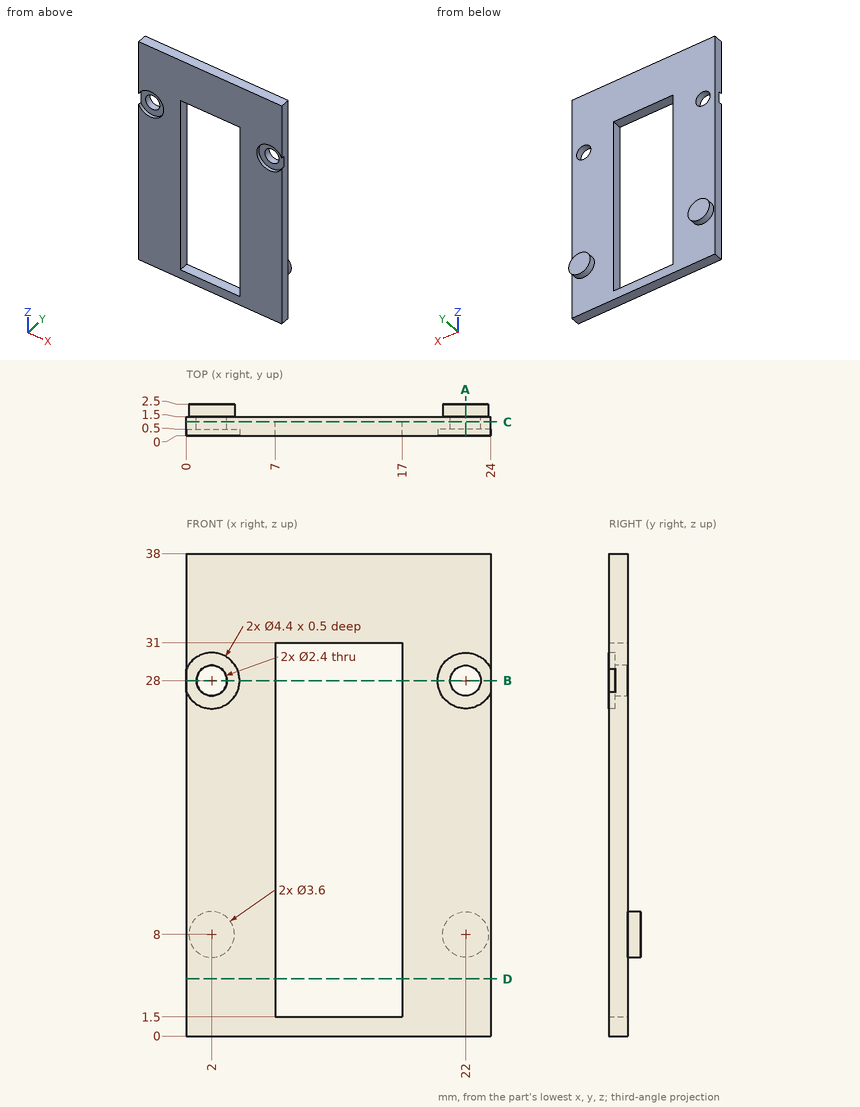
Design review of the part shown in the three views and the two pictorial views. Dimensions are in mm from the part's minimum x, y and z. Give positions to 0.01 mm unless a question says otherwise; leave off trailing zeros. Loops run counter-clockwise (first coordinate to the right, second up) from the corner with the lowest first, then second, coordinate; pieces in that order, holes last. Notation, with made-up numbers: (-32, 54) -> (20, 54) arc R27 ccw to (20, 87) -> close; hole circle Ø6 at (-11.75, 79). An arc over 180 degrees is marked (long way). Answer as a JSON object with one key per item and string values. Group by question number.
Q1. Wall thickness on line 1 along Z through (x, y) = (2, 0.4); line 2 along Z through (x, y) = (12.75, 0.1); line 3 along X through (y, z) = (0.4, 2): over which ranges is each line inside the solid? List them lowest first.
Q2. Take a section at D-D (z = 4.5). Write out the cut boundary in (x, y).
Q3. Insertion check: pin 1 (5 mm diameter, centred on x = 2, z = 28, fed in from +Y); pin 2 (1.2 mm diameter, centred on x = 12.5, y = 1, fed in from -Z); pin 3 (1.3 mm diameter, centred on x = 21.5, z = 27.5, fed in from -Y). Each pin has a flat end and moves straight along its axis. Give the tip position at first contact, or say it passes through.
Q4. Take a section at B-B (z = 28). Write out the cut boundary in (x, y), plus the area to 3 significant figures.
Q5. Take a section at C-C (y = 1.1). Write out the cut boundary in (x, z), plus the area to 3 significant figures.
Q6. Take a section at A-A (x = 22). Write out the cut boundary in (y, z).
Answer below:
{
 "1": {"line 1": "z = 0 to 25.8, 30.2 to 38", "line 2": "z = 0 to 1.5, 31 to 38", "line 3": "x = 0 to 7, 17 to 24"},
 "2": {"outline": "(0, 0) -> (7, 0) -> (7, 1.5) -> (0, 1.5) -> close; (17, 0) -> (24, 0) -> (24, 1.5) -> (17, 1.5) -> close"},
 "3": {"pin 1": "stops at y = 1.5", "pin 2": "stops at z = 0", "pin 3": "stops at y = 0.5"},
 "4": {"outline": "(0, 0.5) -> (0.8, 0.5) -> (0.8, 1.5) -> (0, 1.5) -> close; (3.2, 0.5) -> (4.2, 0.5) -> (4.2, 0) -> (7, 0) -> (7, 1.5) -> (3.2, 1.5) -> close; (17, 0) -> (19.8, 0) -> (19.8, 0.5) -> (20.8, 0.5) -> (20.8, 1.5) -> (17, 1.5) -> close; (23.2, 0.5) -> (24, 0.5) -> (24, 1.5) -> (23.2, 1.5) -> close", "area": "12.0 mm2"},
 "5": {"outline": "(0, 0) -> (24, 0) -> (24, 38) -> (0, 38) -> close; hole circle Ø2.4 at (2, 28); hole (7, 1.5) -> (17, 1.5) -> (17, 31) -> (7, 31) -> close; hole circle Ø2.4 at (22, 28)", "area": "608 mm2"},
 "6": {"outline": "(0, 0) -> (1.5, 0) -> (1.5, 6.2) -> (2.5, 6.2) -> (2.5, 9.8) -> (1.5, 9.8) -> (1.5, 26.8) -> (0.5, 26.8) -> (0.5, 25.8) -> (0, 25.8) -> close; (0, 30.2) -> (0.5, 30.2) -> (0.5, 29.2) -> (1.5, 29.2) -> (1.5, 38) -> (0, 38) -> close"}
}
